Geometry: final body of the model. Coordinates: model frame, mm. Coordinates: 2 decimals unless noted, no trailing zeros. Loops run counter-clockwise (first coordinate to the right, second up) from the corner with the lowest first, then second, coordinate; pieces in that order, holes last. Notation, with made-up numbers: (70.5, 19.25) -> (88.5, 19.25) arc R30 ccw to (88.5, 43.25) -> close; hole circle Ø2 at (31, 61). An arc over 180 degrees is marked (long way). One line per item, written item: value. Start each with the question number.
Item 1: Section query B-B on z = -33. Return loops of the section in (x, y).
Item 2: Section query D-D on x = 103.5. Return loops of the section in (y, z), then the cut area to 3 significant figures.
Item 3: Ray query, probe 1 along X at (y, z) = (1.4, -133); probe 2 along X at (y, z) = (2.7, -88); probe 3 along Z at (x, y) = (-141, 0.9). Return the intervals inside material, ascending. Write a range as from..to.
Item 4: Mould query, pull axis Z, two halves, no side actions, for faces 1 (the flat face through (26, 0, 29)), 2 (the cylindrical face through (-97.129, 2.028, 67.518)), 3 (the cylindrical face through (96.52, 2.03, 52.46)). Classes: +Z half, -Z half, draft (parallel to the pull), parting line (faces both ways), or undercut.
Item 5: Section query C-C on z = -4. Return loops of the section in (x, y).
Item 6: Contact query for flat-ended pins moving along their axis: pin 1 Ø1.2 at (y, z) = (3, 123) entering from -X; pin 2 Ø1.2 at (x, y) = (130, 3) entering from +Z. Output: stop coordinate, or through.
Item 7: Section query A-A on x = -44. Return loops of the section in (y, z).
from build123d import *

# Parameters (mm, degrees)
EXTRUDE_1_DEPTH          = 4
CUT_EXTRUDE_2_DEPTH      = 204.764570031
CUT_EXTRUDE_2_DEPTH_BACK = 204.764570031
SKETCH_3_R               = 2
SKETCH_3_R_2             = 2.297041363
SKETCH_4_R               = 55
CUT_EXTRUDE_3_DEPTH      = 10
SKETCH_5_R               = 2
SKETCH_5_R_2             = 2.1
CUT_EXTRUDE_4_DEPTH      = 204.764570031
SKETCH_6_R               = 1.5
CUT_EXTRUDE_5_DEPTH      = 204.764570031
CUT_EXTRUDE_6_DEPTH      = 204.764570031
CUT_EXTRUDE_7_DEPTH      = 204.764570031
CUT_EXTRUDE_7_DEPTH_BACK = 204.764570031
SKETCH_8_W               = 73
SKETCH_8_H               = 136
CUT_EXTRUDE_8_DEPTH      = 204.764570031
CUT_EXTRUDE_8_DEPTH_BACK = 204.764570031
SKETCH_9_R               = 1.5
SKETCH_9_R_2             = 1.441079752
FILLET_1_R               = 2
FILLET_2_R               = 25
FILLET_3_R               = 25


with BuildPart() as part:
    # 草图1 → 凸台-拉伸1 (new body)
    with BuildSketch(Plane(origin=(0, 0, 0), x_dir=(1, 0, 0), z_dir=(0, 1, 0))):
        Polygon((-90, -140), (90, -140), (90, -60), (140, -60), (140, 60), (90, 60), (90, 140), (-90, 140), (-90, 60), (-140, 60), (-148, 60), (-148, -60), (-140, -60), (-90, -60), align=None)
    extrude(amount=EXTRUDE_1_DEPTH)

    # 草图3 → 切除-拉伸2 (cut, two sides: drawn at the far end of the back side and taken through both)
    with BuildSketch(Plane(origin=(0, 4, 0), x_dir=(1, 0, 0), z_dir=(0, 1, 0)).offset(-CUT_EXTRUDE_2_DEPTH_BACK)):
        with Locations(Location((-83, -133, 0), (0, 0, 270))):
            Circle(SKETCH_3_R)
        with Locations(Location((83, -133, 0), (0, 0, 270))):
            Circle(SKETCH_3_R)
        with Locations(Location((-83, 133, 0), (0, 0, 270))):
            Circle(SKETCH_3_R)
        with Locations(Location((83, 133, 0), (0, 0, 270))):
            Circle(SKETCH_3_R)
        with Locations(Location((133, 53, 0), (0, 0, 270))):
            Circle(SKETCH_3_R)
        with Locations(Location((133, -53, 0), (0, 0, 270))):
            Circle(SKETCH_3_R)
        with Locations(Location((32.977399051, 47.022600949, 0), (0, 0, 270))):
            Circle(SKETCH_3_R)
        with Locations(Location((127.022600949, 47.022600949, 0), (0, 0, 270))):
            Circle(SKETCH_3_R)
        with Locations(Location((127.022600949, -47.022600949, 0), (0, 0, 270))):
            Circle(SKETCH_3_R)
        with Locations(Location((32.977399051, -47.022600949, 0), (0, 0, 270))):
            Circle(SKETCH_3_R)
        with Locations(Location((-141, 53, 0), (0, 0, 270))):
            Circle(SKETCH_3_R_2)
        with Locations(Location((-141, -53, 0), (0, 0, 270))):
            Circle(SKETCH_3_R)
        with Locations(Location((20, -53, 0), (0, 0, 270))):
            Circle(SKETCH_3_R)
        with Locations(Location((20, 53, 0), (0, 0, 270))):
            Circle(SKETCH_3_R)
        with Locations(Location((-81, 53, 0), (0, 0, 270))):
            Circle(SKETCH_3_R)
        with Locations(Location((-81, -53, 0), (0, 0, 270))):
            Circle(SKETCH_3_R)
        with Locations(Location((70, -73.854225456, 0), (0, 0, 270))):
            Circle(SKETCH_3_R)
        with Locations(Location((2, -133, 0), (0, 0, 270))):
            Circle(SKETCH_3_R)
    extrude(amount=CUT_EXTRUDE_2_DEPTH + CUT_EXTRUDE_2_DEPTH_BACK, mode=Mode.SUBTRACT)

    # 草图4 → 切除-拉伸3 (cut)
    with BuildSketch(Plane(origin=(0, 4, 0), x_dir=(1, 0, 0), z_dir=(0, 1, 0))):
        with Locations(Location((80, 0, 0), (0, 0, 270))):
            Circle(SKETCH_4_R)
    extrude(amount=-CUT_EXTRUDE_3_DEPTH, mode=Mode.SUBTRACT)

    # 草图5 → 切除-拉伸4 (cut, through all)
    with BuildSketch(Plane(origin=(0, 4, 0), x_dir=(1, 0, 0), z_dir=(0, 1, 0))):
        with Locations(Location((-110.053769942, 14.625081272, 0), (0, 0, 270))):
            Circle(SKETCH_5_R)
        with Locations(Location((-120.053769942, 14.625081272, 0), (0, 0, 270))):
            Circle(SKETCH_5_R)
        with Locations(Location((-120.053769942, -35.374918728, 0), (0, 0, 270))):
            Circle(SKETCH_5_R_2)
        with Locations(Location((-109.860583636, -35.374918728, 0), (0, 0, 270))):
            Circle(SKETCH_5_R_2)
        Polygon((-105.053769942, 9.625081272), (-105.053769942, -30.374918728), (-114.053769942, -30.374918728), (-114.053769942, -35.874918728), (-114.553769942, -36.374918728), (-115.553769942, -36.374918728), (-116.053769942, -35.874918728), (-116.053769942, -30.374918728), (-125.053769942, -30.374918728), (-125.053769942, 9.625081272), (-116.053769942, 9.625081272), (-116.053769942, 15.125081272), (-115.553769942, 15.625081272), (-114.553769942, 15.625081272), (-114.053769942, 15.125081272), (-114.053769942, 9.625081272), align=None)
    extrude(amount=-CUT_EXTRUDE_4_DEPTH, mode=Mode.SUBTRACT)

    # 草图6 → 切除-拉伸5 (cut, through all)
    with BuildSketch(Plane(origin=(0, 4, 0), x_dir=(1, 0, 0), z_dir=(0, 1, 0))):
        with Locations(Location((40, -122, 0), (0, 0, 270))):
            Circle(SKETCH_6_R)
        with Locations(Location((40, -70, 0), (0, 0, 270))):
            Circle(SKETCH_6_R)
        with Locations(Location((-59, -122, 0), (0, 0, 270))):
            Circle(SKETCH_6_R)
        with Locations(Location((-59, -70, 0), (0, 0, 270))):
            Circle(SKETCH_6_R)
    extrude(amount=-CUT_EXTRUDE_5_DEPTH, mode=Mode.SUBTRACT)

    # 草图7 → 切除-拉伸6 (cut, through all)
    with BuildSketch(Plane(origin=(0, 4, 0), x_dir=(1, 0, 0), z_dir=(0, 1, 0))):
        with BuildLine():
            Line((82, -110.6), (52, -110.6))
            ThreePointArc((52, -110.6), (49.9, -108.5), (52, -106.4))
            Line((52, -106.4), (82, -106.4))
            ThreePointArc((82, -106.4), (84.1, -108.5), (82, -110.6))
        make_face()
        with BuildLine():
            Line((82, -85.6), (52, -85.6))
            ThreePointArc((52, -85.6), (49.9, -83.5), (52, -81.4))
            Line((52, -81.4), (82, -81.4))
            ThreePointArc((82, -81.4), (84.1, -83.5), (82, -85.6))
        make_face()
    extrude(amount=-CUT_EXTRUDE_6_DEPTH, mode=Mode.SUBTRACT)

    # 草图8 → 切除-拉伸7 (cut, two sides: drawn at the far end of the back side and taken through both)
    with BuildSketch(Plane(origin=(0, 4, 0), x_dir=(1, 0, 0), z_dir=(0, 1, 0)).offset(-CUT_EXTRUDE_7_DEPTH_BACK)):
        with Locations((-28, 7)):
            Rectangle(SKETCH_8_W, SKETCH_8_H)
    extrude(amount=CUT_EXTRUDE_7_DEPTH + CUT_EXTRUDE_7_DEPTH_BACK, mode=Mode.SUBTRACT)

    # 草图9 → 切除-拉伸8 (cut, two sides: drawn at the far end of the back side and taken through both)
    with BuildSketch(Plane(origin=(0, 4, 0), x_dir=(1, 0, 0), z_dir=(0, 1, 0)).offset(-CUT_EXTRUDE_8_DEPTH_BACK)):
        with Locations(Location((-51.339528663, 88, 0), (0, 0, 270))):
            Circle(SKETCH_9_R)
        with Locations(Location((-51.339528663, 130, 0), (0, 0, 270))):
            Circle(SKETCH_9_R)
        with Locations(Location((32.160471337, 130, 0), (0, 0, 270))):
            Circle(SKETCH_9_R_2)
        with Locations(Location((32.160471337, 88, 0), (0, 0, 270))):
            Circle(SKETCH_9_R)
    extrude(amount=CUT_EXTRUDE_8_DEPTH + CUT_EXTRUDE_8_DEPTH_BACK, mode=Mode.SUBTRACT)

    # 圆角1
    fillet_1_edges = [part.edges().sort_by_distance(p)[0] for p in [
        (-148, 2, -60),
        (-90, 2, -140),
        (90, 2, -140),
        (140, 2, -60),
        (140, 2, 60),
        (90, 2, 140),
        (-90, 2, 140),
        (-148, 2, 60),
    ]]
    fillet(fillet_1_edges, radius=FILLET_1_R)

    # 圆角2
    fillet_2_edges = [part.edges().sort_by_distance(p)[0] for p in [
        (-90, 2, 60),
    ]]
    fillet(fillet_2_edges, radius=FILLET_2_R)

    # 圆角3
    fillet_3_edges = [part.edges().sort_by_distance(p)[0] for p in [
        (-90, 2, -60),
        (90, 2, -60),
        (90, 2, 60),
    ]]
    fillet(fillet_3_edges, radius=FILLET_3_R)


solid = part.part
Reply:
1. outline: (-148, 0) -> (-64.5, 0) -> (-64.5, 4) -> (-148, 4) -> close; (8.5, 0) -> (36, 0) -> (36, 4) -> (8.5, 4) -> close; (124, 0) -> (140, 0) -> (140, 4) -> (124, 4) -> close
2. outline: (0, -62.8) -> (4, -62.8) -> (4, -49.73) -> (0, -49.73) -> close; (0, 49.73) -> (4, 49.73) -> (4, 62.8) -> (0, 62.8) -> close
2. area: 105 mm²
3. probe 1: x = -90..-85, -81..81, 85..90
3. probe 2: x = -90..-52.84, -49.84..30.66, 33.66..90
3. probe 3: z = -60..-55.3, -50.7..51, 55..60
4. face 1: draft
4. face 2: +Z half
4. face 3: undercut
5. outline: (-148, 0) -> (-125.05, 0) -> (-125.05, 4) -> (-148, 4) -> close; (-105.05, 0) -> (-64.5, 0) -> (-64.5, 4) -> (-105.05, 4) -> close; (8.5, 0) -> (25.15, 0) -> (25.15, 4) -> (8.5, 4) -> close; (134.85, 0) -> (140, 0) -> (140, 4) -> (134.85, 4) -> close
6. pin 1: stops at x = -90
6. pin 2: stops at z = 60
7. outline: (0, -140) -> (4, -140) -> (4, -75) -> (0, -75) -> close; (0, 61) -> (4, 61) -> (4, 140) -> (0, 140) -> close
